The drawing under review shows one solid part. Ordinate dimensions are in mm from its lowest x, y, z. A direction names the side the tool comes from. Round coordinates to 2 decimals unless told otherwise and drop trailing zeros. Order: outer loops, then holes, each group sorted by start corner. A loop starts at its lowest first (then second) coordinate and runs counter-clockwise, first axis right, second up.
1) Consider section A-A (x = 4). Give the boundary of the cut face in (y, z).
2) Clearance check with flat-ended pins moving along their axes: P1, Ø2, axis at y = 11.5, z = 6.5, coming from the -X side; P2, Ø3, axis at x = 1, y = 15, coming from the -Z side; P3, Ø1.5, axis at y = 10.5, z = 2.5, coming from the +X side. State where each tip first meets the part, or that it passes through.
3) Consider section B-B (z = 4). Give the boundary of the cut face in (x, y), then the cut area to 3 significant figures.
4) Machinability: for the marked faces 1 and 2, which of the approach directions +Z, -Z, +X, -X, +Y, -Y give a long, thin tool a straight path to every point of the face, cutting with its end or side? Answer none if there is none.
5) To check wall thickness, follow L1, parallel to Y at x = 5.5, z = 7.25; L2, parallel to X at y = 5.25, z = 4; L3, parallel to X at y = 10.5, z = 4.5. State the ranges of each line that lie inside material, in increasing order.
6) Consider section C-C (y = 23). Give the boundary of the cut face in (x, z), then the cut area to 3 significant figures.
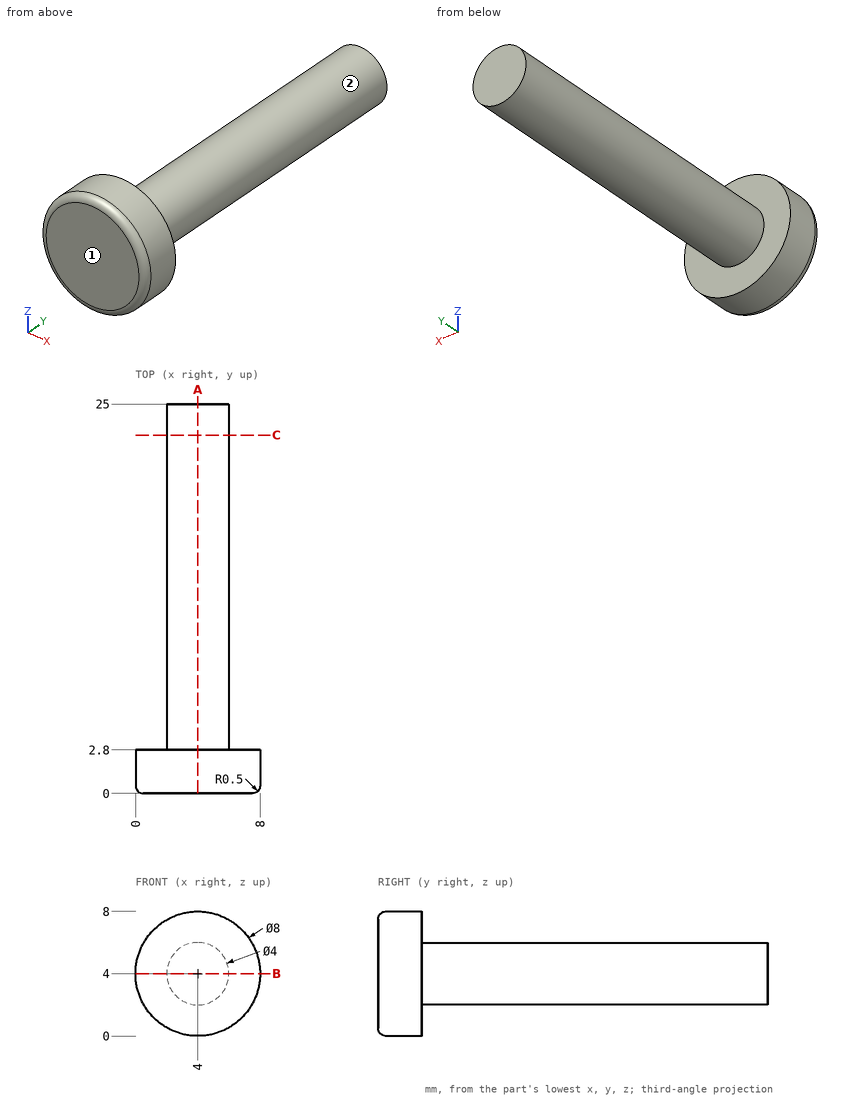
Answer below:
1. outline: (0, 0.5) arc R0.5 ccw to (0.5, 0) - (2.8, 0) - (2.8, 2) - (25, 2) - (25, 6) - (2.8, 6) - (2.8, 8) - (0.5, 8) arc R0.5 ccw to (0, 7.5) - close
2. P1: stops at x = 2.68
2. P2: stops at z = 2.68
2. P3: stops at x = 5.85
3. outline: (0, 0.5) arc R0.5 ccw to (0.5, 0) - (7.5, 0) arc R0.5 ccw to (8, 0.5) - (8, 2.8) - (6, 2.8) - (6, 25) - (2, 25) - (2, 2.8) - (0, 2.8) - close
3. area: 111 mm2
4. face 1: +Z, -Z, +X, -X, -Y
4. face 2: +Y
5. L1: y = 0.01 to 2.8
5. L2: x = 2 to 6
5. L3: x = 2.06 to 5.94
6. outline: circle Ø4 at (4, 4)
6. area: 12.6 mm2
